Could you check a few things on this model? Use its own coordinates, in mm. A direction names the side the tool comes from. Coordinates: 2 decimals unless noted, no trailing zeros. Order: outer loops, then holes, each group sorted by start corner. A loop starts at its lowest first (then second) coordinate and runs counter-clockwise, first axis right, second up. Notation, with made-up numbers: (43, 70.5) - (60, 70.5) arc R23 cw to (60, 97.5) - close; hole circle Ø7 at (3.5, 42). An arc over 180 degrees is marked (long way). One line per item, written item: value. Start each with the question number.
from build123d import *

# Parameters (mm, degrees)
SKETCH1_W           = 26
SKETCH1_H           = 26
BOSS_EXTRUDE1_DEPTH = 250
SHELL1_T            = -3
SKETCH2_W           = 10
SKETCH2_H           = 244
CUT_EXTRUDE1_DEPTH  = 3
CHAMFER1_SIZE       = 0.3


with BuildPart() as part:
    # Sketch1 → Boss-Extrude1 (new body)
    with BuildSketch(Plane(origin=(0, 0, 0), x_dir=(1, 0, 0), z_dir=(0, 1, 0))):
        Rectangle(SKETCH1_W, SKETCH1_H)
    extrude(amount=BOSS_EXTRUDE1_DEPTH)

    # Shell1
    shell1_openings = [part.faces().sort_by_distance(p)[0] for p in [
        (0, 250, 0),
        (0, 0, 0),
    ]]
    offset(amount=SHELL1_T, openings=shell1_openings, kind=Kind.INTERSECTION)

    # Sketch2 → Cut-Extrude1 (cut)
    with BuildSketch(Plane.XY.offset(13)):
        with Locations((0, 125)):
            Rectangle(SKETCH2_W, SKETCH2_H)
    extrude(amount=-CUT_EXTRUDE1_DEPTH, mode=Mode.SUBTRACT)

    # Chamfer1
    chamfer1_edges = [part.edges().sort_by_distance(p)[0] for p in [
        (10, 125, 10),
        (13, 125, 13),
        (-13, 125, 13),
        (13, 125, -13),
    ]]
    chamfer(chamfer1_edges, length=CHAMFER1_SIZE)


solid = part.part
Q1. I want a section at C-C on y = 127. Please give me the cut outline in (x, z), then the cut area to 3 significant figures.
Q2. I want a section at A-A on x = 7.5. Please give me the cut outline in (y, z).
Q3. I want a section at B-B on z = -3.5. Please give me the cut outline in (x, y), then the cut area to 3 significant figures.
Q4. We'd pull the mould along X, two halves only. Please class faces 3 (the flat face through (13, 123, 0)), 4 (the flat face through (0, 123, -13)), 5 (the flat face through (10, 123, 0)), 6 (the flat face through (-13, 123, 0)): +X half, -X half, draft (parallel to the pull), parting line (faces both ways), or undercut.
Q5. Which directions (+Z, -Z, +X, -X, +Y, -Y) give clear straight access to the entire face, cutting with the end or side of a thin tool? Please do faces 1 (the flat face through (-12, 0, 0)), 2 (the flat face through (0, 123, -10)).
Q6. If I drill on L1, parallel to X at y = 178.5, z = 3.75; L2, parallel to X at y = 62, z = 10.75, over which ranges is the centre line in solid material (lowest first)?
Q7. I'm going to push a flat-ended pin straight in: pin 1 (5 mm diameter, centred on x = 5.5, z = 6, fed in from -Y). Where does the tip first touch, or does it pass through?
Values follow:
1. outline: (-13, -13) - (12.7, -13) - (13, -12.7) - (13, 12.7) - (12.7, 13) - (5, 13) - (5, 10) - (9.7, 10) - (10, 9.7) - (10, -10) - (-10, -10) - (-10, 10) - (-5, 10) - (-5, 13) - (-12.7, 13) - (-13, 12.7) - close
1. area: 246 mm^2
2. outline: (0, -13) - (250, -13) - (250, -10) - (0, -10) - close; (0, 10) - (250, 10) - (250, 13) - (0, 13) - close
3. outline: (-13, 0) - (-10, 0) - (-10, 250) - (-13, 250) - close; (10, 0) - (13, 0) - (13, 250) - (10, 250) - close
3. area: 1,500 mm^2
4. face 3: +X half
4. face 4: draft
4. face 5: undercut
4. face 6: -X half
5. face 1: +Z, -Z, +X, -X, -Y
5. face 2: +Y, -Y
6. L1: x = -13 to -10, 10 to 13
6. L2: x = -13 to -5, 5 to 13
7. pin 1: passes through
